Work out the finished part from the listing and answer in its coordinate system (mm). Face numbers are marked on the shaded views. A direction names the side the tool comes from. Coordinates: 2 decimals unless noted, no trailing zeros. Order: outer loops, then holes, each group sorted by start corner. A loop starts at its lowest first (then second) coordinate and runs counter-clockwise, first axis right, second up.
```python
from build123d import *

# Parameters (mm, degrees)
F1_DEPTH  = 2
F3_DEPTH  = 8
F5_DEPTH  = 2
F7_DEPTH  = 5
F9_DEPTH  = 2
F11_DEPTH = 10
F12_R     = 1.5
F13_DEPTH = 12.001


with BuildPart() as f1:
    # F0 (on Front) → F1 (new body)
    with BuildSketch(Plane.XZ):
        with BuildLine():
            ThreePointArc((20.9852738604, 27.6129976553), (6.6475053794, 16.5350086475), (-2.8008963523, 1.074699783))
            ThreePointArc((-2.8008963523, 1.074699783), (-1.7031308032, -2.4696852972), (2, -2.2360679775))
            ThreePointArc((2, -2.2360679775), (12, 1.583592135), (22, -2.2360679775))
            ThreePointArc((22, -2.2360679775), (25.8098712045, -2.3925647793), (26.6958733889, 1.3161560208))
            ThreePointArc((26.6958733889, 1.3161560208), (23.7193066232, 12.5085096075), (25.2040552071, 23.994337839))
            ThreePointArc((25.2040552071, 23.994337839), (24.3121710173, 27.2230865107), (20.9852738604, 27.6129976553))
        make_face()
    extrude(amount=F1_DEPTH)

    # F2 (on face) → F3 (join)
    with BuildSketch(Plane.XZ.offset(2)):
        with BuildLine():
            ThreePointArc((2.1819579837, 4.4987842088), (3.4387063042, 3.6297794635), (4.3743364575, 2.4218134851))
            ThreePointArc((4.3743364575, 2.4218134851), (5.8533522977, 1.1022435306), (7.83244861, 0.9930166694))
            ThreePointArc((7.83244861, 0.9930166694), (11.5712509604, 1.5774633583), (15.3373412263, 1.2076187193))
            ThreePointArc((15.3373412263, 1.2076187193), (17.2681996472, 1.4114232526), (18.6698729811, 2.7549493575))
            ThreePointArc((18.6698729811, 2.7549493575), (20.1092125836, 4.5674690235), (22.1275149749, 5.7003333087))
            ThreePointArc((22.1275149749, 5.7003333087), (23.7699182337, 7.0173378758), (24.1424847183, 9.0893378054))
            ThreePointArc((24.1424847183, 9.0893378054), (23.7937370176, 11.591814757), (23.6568029492, 14.1147624204))
            ThreePointArc((23.6568029492, 14.1147624204), (22.9247140991, 16.0425380377), (21.1211981937, 17.0423396652))
            ThreePointArc((21.1211981937, 17.0423396652), (18.064820066, 18.1961838029), (15.724550358, 20.475644539))
            ThreePointArc((15.724550358, 20.475644539), (13.6368998786, 21.7724389046), (11.2806267778, 21.0739138692))
            ThreePointArc((11.2806267778, 21.0739138692), (5.5962553568, 15.3235804079), (0.9130746838, 8.7322048192))
            ThreePointArc((0.9130746838, 8.7322048192), (0.6174404831, 6.3367228484), (2.1819579837, 4.4987842088))
        make_face()
    extrude(amount=F3_DEPTH)

    # F4 (on face) → F5 (join)
    with BuildSketch(Plane.XZ.offset(2)):
        with BuildLine():
            ThreePointArc((2, -2.2360679775), (4.7345595446, -0.2933984926), (7.83244861, 0.9930166694))
            ThreePointArc((7.83244861, 0.9930166694), (5.8533522977, 1.1022435306), (4.3743364575, 2.4218134851))
            ThreePointArc((4.3743364575, 2.4218134851), (3.4387063042, 3.6297794635), (2.1819579837, 4.4987842088))
            ThreePointArc((2.1819579837, 4.4987842088), (0.6174404831, 6.3367228484), (0.9130746838, 8.7322048192))
            ThreePointArc((0.9130746838, 8.7322048192), (-1.1071325681, 4.9826165706), (-2.8008963523, 1.074699783))
            ThreePointArc((-2.8008963523, 1.074699783), (-1.7031308032, -2.4696852972), (2, -2.2360679775))
        make_face()
    extrude(amount=F5_DEPTH)

    # F6 (on face) → F7 (join)
    with BuildSketch(Plane.XZ.offset(2)):
        with BuildLine():
            ThreePointArc((26.6958733889, 1.3161560208), (25.1529407341, 5.1152911032), (24.1424847183, 9.0893378054))
            ThreePointArc((24.1424847183, 9.0893378054), (23.7699182337, 7.0173378758), (22.1275149749, 5.7003333087))
            ThreePointArc((22.1275149749, 5.7003333087), (20.1092125836, 4.5674690235), (18.6698729811, 2.7549493575))
            ThreePointArc((18.6698729811, 2.7549493575), (17.2681996472, 1.4114232526), (15.3373412263, 1.2076187193))
            ThreePointArc((15.3373412263, 1.2076187193), (18.8873733936, -0.0910903177), (22, -2.2360679775))
            ThreePointArc((22, -2.2360679775), (25.8098712045, -2.3925647793), (26.6958733889, 1.3161560208))
        make_face()
    extrude(amount=F7_DEPTH)

    # F8 (on face) → F9 (join)
    with BuildSketch(Plane.XZ.offset(10)):
        with BuildLine():
            ThreePointArc((17.7815184779, 3.2141075837), (19.4607480142, 5.3287138608), (21.8154341374, 6.6503888602))
            ThreePointArc((21.8154341374, 6.6503888602), (22.9103696432, 7.5283919049), (23.1587472996, 8.9097251913))
            ThreePointArc((23.1587472996, 8.9097251913), (22.7983746756, 11.4956180412), (22.6568761383, 14.1026639602))
            ThreePointArc((22.6568761383, 14.1026639602), (22.1688169049, 15.387847705), (20.966472968, 16.0543821233))
            ThreePointArc((20.966472968, 16.0543821233), (17.5280475743, 17.3524567782), (14.8952441528, 19.9168501063))
            ThreePointArc((14.8952441528, 19.9168501063), (13.5034771665, 20.7813796834), (11.9326284326, 20.3156963265))
            ThreePointArc((11.9326284326, 20.3156963265), (6.3619444401, 14.6803695344), (1.7724273805, 8.2208214575))
            ThreePointArc((1.7724273805, 8.2208214575), (1.5753379134, 6.623833477), (2.6183495805, 5.3985410505))
            ThreePointArc((2.6183495805, 5.3985410505), (4.1264475651, 4.3557353562), (5.249203749, 2.9061761822))
            ThreePointArc((5.249203749, 2.9061761822), (6.2352143091, 2.0264628791), (7.5546118506, 1.9536449717))
            ThreePointArc((7.5546118506, 1.9536449717), (11.5426676911, 2.5770547732), (15.5598306414, 2.1825538249))
            ThreePointArc((15.5598306414, 2.1825538249), (16.8470695887, 2.3184235138), (17.7815184779, 3.2141075837))
        make_face()
    extrude(amount=F9_DEPTH)

    # F10 (on face) → F11 (cut)
    with BuildSketch(Plane.XZ.offset(12)):
        with BuildLine():
            ThreePointArc((14.0659379899, 19.3580557023), (13.3700544612, 19.7903205129), (12.5846300541, 19.5574788225))
            ThreePointArc((12.5846300541, 19.5574788225), (7.1276334842, 14.0371586938), (2.6317800333, 7.7094381219))
            ThreePointArc((2.6317800333, 7.7094381219), (2.5332352947, 6.9109440908), (3.0547411549, 6.2982978463))
            ThreePointArc((3.0547411549, 6.2982978463), (4.8141887907, 5.0816912117), (6.1240709957, 3.3905388544))
            ThreePointArc((6.1240709957, 3.3905388544), (6.617076301, 2.9506821804), (7.2767751055, 2.9142732248))
            ThreePointArc((7.2767751055, 2.9142732248), (11.5140844233, 3.576646137), (15.7823200452, 3.1574888807))
            ThreePointArc((15.7823200452, 3.1574888807), (16.4259395517, 3.2254237286), (16.8931640202, 3.6732657865))
            ThreePointArc((16.8931640202, 3.6732657865), (18.812283478, 6.0899586591), (21.5033533158, 7.6004443631))
            ThreePointArc((21.5033533158, 7.6004443631), (22.0508210967, 8.0394459079), (22.1750099313, 8.7301125864))
            ThreePointArc((22.1750099313, 8.7301125864), (21.8030123845, 11.3994213304), (21.6569493785, 14.0905655005))
            ThreePointArc((21.6569493785, 14.0905655005), (21.4129197493, 14.7331574058), (20.8117477501, 15.066424632))
            ThreePointArc((20.8117477501, 15.066424632), (16.99127511, 16.5087297967), (14.0659379899, 19.3580557023))
        make_face()
    extrude(amount=-F11_DEPTH, mode=Mode.SUBTRACT)

    # F12 (on Front) → F13 (cut, through all)
    with BuildSketch(Plane.XZ):
        Circle(F12_R)
        with Locations((22.359, 24.946)):
            Circle(F12_R)
        with Locations((24, 0)):
            Circle(F12_R)
    extrude(amount=F13_DEPTH, mode=Mode.SUBTRACT)


solid = f1.part
```
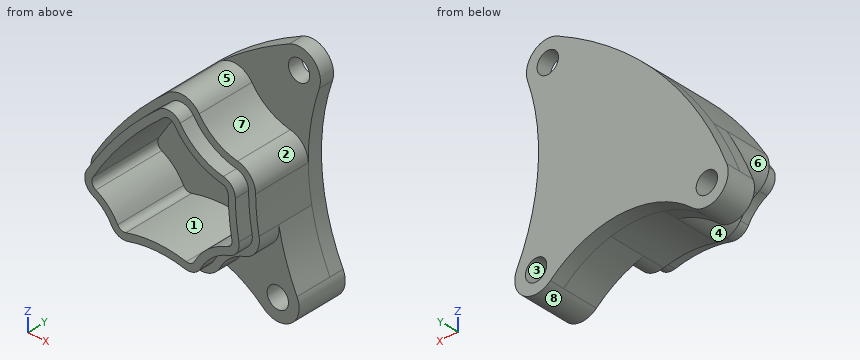
1. The part is cut by section C-C (x = 20). Determine the outline of the cut face in (y, z), plus the area to 3 significant figures.
2. Flat-ended cylindrical pins translate along their axes: pin 1 (1.5 mm diameter, centred on y = -9, z = 15.5, fed in from +X); pin 2 (1.5 mm diameter, centred on x = 6.5, y = -3.5, fed in from -Z); pin 3 (8 mm diameter, centred on x = 22.5, z = 21, fed in from -Y); pin 4 (2.5 mm diameter, centred on x = 22.359, z = 24.946, fed in from +Y). Find the tip coordinate at first contact, or state that the pin passes through.
3. Consider probe 1 along Z at (x, y) = (23, -1.5); probe 2 along Y at (x, z) = (7.75, 14.5); probe 3 along X at (y, z) = (-0.85, 0). Determine where each line is inside the solid, lowest interval first.
4. The mould has two halves that part along X. Classify the marked faces 5, 6, 7 and 8: released by +X, released by -X, zero draft, split by the parting line, or undercut.
5. The part is cut by section D-D (y = -5). Determine the outline of the cut face in (x, z) (1 decimal), plus the area to 3 significant figures.
6. The part is cut by section B-B (z = 0). Determine the outline of the cut face in (x, y).
7. For the marked faces 1, 2, 3 and 4, determine the directions among +Z, -Z, +X, -X, +Y, -Y from which every point of the face is accessible in a straight line to the end or side of a thin tool.
8. The part is cut by section A-A (x = 0). Determine the outline of the cut face in (y, z).
Worked out:
1. outline: (-12, 5.74) - (-10, 5.74) - (-10, 4.47) - (-7, 4.47) - (-7, -0.73) - (0, -0.73) - (0, 27.09) - (-2, 27.09) - (-2, 17.3) - (-10, 17.3) - (-10, 16.26) - (-12, 16.26) - (-12, 15.23) - (-2, 15.23) - (-2, 6.93) - (-12, 6.93) - close
1. area: 122 mm2
2. pin 1: stops at x = 23.58
2. pin 2: stops at z = 0.22
2. pin 3: stops at y = -2
2. pin 4: passes through
3. probe 1: z = -2.83 to -1.12, 1.12 to 23.59, 26.3 to 27.88
3. probe 2: y = -2 to 0
3. probe 3: x = -3 to -1.5, 1.5 to 5.29, 18.71 to 22.5, 25.5 to 27
4. face 5: split by the parting line
4. face 6: released by -X
4. face 7: released by +X
4. face 8: undercut
5. outline: (0.9, 8.7) arc R3 ccw to (2.2, 4.5) arc R5 cw to (4.4, 2.4) arc R3 ccw to (7.8, 1) arc R15 cw to (22, -2.2) arc R3 ccw to (26.7, 1.3) arc R30 cw to (23.7, 14.1) arc R3 ccw to (21.1, 17) arc R8 cw to (15.7, 20.5) arc R3 ccw to (11.3, 21.1) arc R50 ccw to start; hole (2.6, 7.7) arc R1 ccw to (3.1, 6.3) arc R7 cw to (6.1, 3.4) arc R1 ccw to (7.3, 2.9) arc R17 cw to (15.8, 3.2) arc R1 ccw to (16.9, 3.7) arc R8 cw to (21.5, 7.6) arc R1 ccw to (22.2, 8.7) arc R32 cw to (21.7, 14.1) arc R1 ccw to (20.8, 15.1) arc R10 cw to (14.1, 19.4) arc R1 ccw to (12.6, 19.6) arc R48 ccw to start; hole circle Ø3 at (24, 0)
5. area: 179 mm2
6. outline: (-3, -4) - (-1.5, -4) - (-1.5, 0) - (-3, 0) - close; (1.5, -4) - (5.29, -4) - (5.29, 0) - (1.5, 0) - close; (18.71, -7) - (22.5, -7) - (22.5, 0) - (18.71, 0) - close; (25.5, -7) - (27, -7) - (27, 0) - (25.5, 0) - close
7. face 1: -Y
7. face 2: +Z, +X, -Y
7. face 3: +Y, -Y
7. face 4: -Z, -Y
8. outline: (-4, -3) - (0, -3) - (0, -1.5) - (-4, -1.5) - close; (-4, 1.5) - (0, 1.5) - (0, 7.13) - (-4, 7.13) - close
